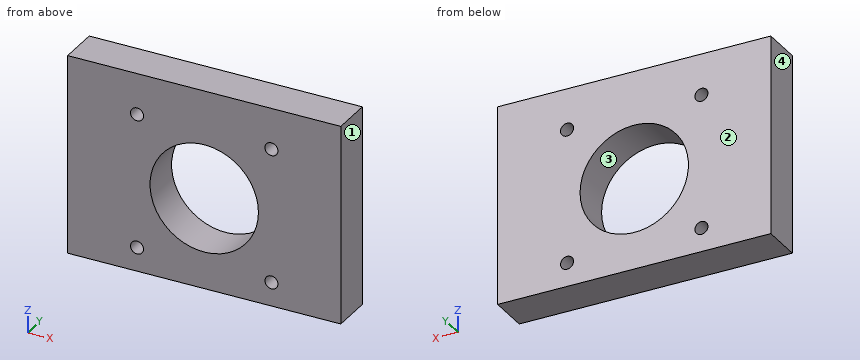
```python
from build123d import *

# Parameters (mm, degrees)
BOSS_EXTRUDE1_DEPTH = 46
CUT_EXTRUDE1_REACH  = 11.3
SKETCH2_R           = 12.5
SKETCH2_R_2         = 1.5


with BuildPart() as part:
    # Sketch1 → Boss-Extrude1 (new body)
    with BuildSketch(Plane.XY):
        Polygon((0, 0), (-31.5, 0), (-31.5, 9.3), (31.5, 9.3), (31.5, 0), align=None)
    extrude(amount=BOSS_EXTRUDE1_DEPTH)

    # Sketch2 → Cut-Extrude1 (cut, up to next)
    with BuildSketch(Plane(origin=(0, 9.3, 0), x_dir=(1, 0, 0), z_dir=(0, 1, 0)), mode=Mode.PRIVATE) as cut_extrude1_sk1:
        with Locations((0, -21)):
            Circle(SKETCH2_R)
    cut_extrude1_tool1 = extrude(cut_extrude1_sk1.sketch, amount=-CUT_EXTRUDE1_REACH, mode=Mode.PRIVATE) & part.part
    add(cut_extrude1_tool1.solids().sort_by_distance((0, 9.3, 21))[0], mode=Mode.SUBTRACT)
    # Sketch2 → Cut-Extrude1 (cut, up to next)
    with BuildSketch(Plane(origin=(0, 9.3, 0), x_dir=(1, 0, 0), z_dir=(0, 1, 0)), mode=Mode.PRIVATE) as cut_extrude1_sk2:
        with Locations((-15.5, -5.5)):
            Circle(SKETCH2_R_2)
    cut_extrude1_tool2 = extrude(cut_extrude1_sk2.sketch, amount=-CUT_EXTRUDE1_REACH, mode=Mode.PRIVATE) & part.part
    add(cut_extrude1_tool2.solids().sort_by_distance((-15.5, 9.3, 5.5))[0], mode=Mode.SUBTRACT)
    # Sketch2 → Cut-Extrude1 (cut, up to next)
    with BuildSketch(Plane(origin=(0, 9.3, 0), x_dir=(1, 0, 0), z_dir=(0, 1, 0)), mode=Mode.PRIVATE) as cut_extrude1_sk3:
        with Locations((-15.5, -36.5)):
            Circle(SKETCH2_R_2)
    cut_extrude1_tool3 = extrude(cut_extrude1_sk3.sketch, amount=-CUT_EXTRUDE1_REACH, mode=Mode.PRIVATE) & part.part
    add(cut_extrude1_tool3.solids().sort_by_distance((-15.5, 9.3, 36.5))[0], mode=Mode.SUBTRACT)
    # Sketch2 → Cut-Extrude1 (cut, up to next)
    with BuildSketch(Plane(origin=(0, 9.3, 0), x_dir=(1, 0, 0), z_dir=(0, 1, 0)), mode=Mode.PRIVATE) as cut_extrude1_sk4:
        with Locations((15.5, -5.5)):
            Circle(SKETCH2_R_2)
    cut_extrude1_tool4 = extrude(cut_extrude1_sk4.sketch, amount=-CUT_EXTRUDE1_REACH, mode=Mode.PRIVATE) & part.part
    add(cut_extrude1_tool4.solids().sort_by_distance((15.5, 9.3, 5.5))[0], mode=Mode.SUBTRACT)
    # Sketch2 → Cut-Extrude1 (cut, up to next)
    with BuildSketch(Plane(origin=(0, 9.3, 0), x_dir=(1, 0, 0), z_dir=(0, 1, 0)), mode=Mode.PRIVATE) as cut_extrude1_sk5:
        with Locations((15.5, -36.5)):
            Circle(SKETCH2_R_2)
    cut_extrude1_tool5 = extrude(cut_extrude1_sk5.sketch, amount=-CUT_EXTRUDE1_REACH, mode=Mode.PRIVATE) & part.part
    add(cut_extrude1_tool5.solids().sort_by_distance((15.5, 9.3, 36.5))[0], mode=Mode.SUBTRACT)


solid = part.part
```
CAD build for the part. Positions are in the model's coordinates, mm. Face numbers are marked on the shaded views. Round coordinates to 2 decimals unless told otherwise and drop trailing zeros. Order: outer loops, then holes, each group sorted by start corner. A loop starts at its lowest first (then second) coordinate and runs counter-clockwise, first axis right, second up.
Q1. Two-plate mould, pull along X, no slides. Class the marked faces 1, 2, 3 and 4: pulls with the +X half, pulls with the -X half, needs draft (parallel to the pull), parting line crosses it, or undercut.
Q2. Slice it at D-D (x = -10.5). Write the cut outline in (y, z).
Q3. Slice it at C-C (y = 2.5). Write the cut outline in (x, z).
Q4. Wall check: L1, parallel to Z at x = -15.5, y = 4.75; L2, parallel to X at y = 4, z = 5.5; L3, parallel to X at y = 4.75, z = 21. Give the ranges that are in metal, low to high.
Q5. Slice it at B-B (z = 5.5). Write the cut outline in (x, y).
Q6. Slice it at A-A (x = 15.5). Write the cut outline in (y, z), and give its area (3 significant figures).
Results below:
1. face 1: pulls with the +X half
1. face 2: needs draft
1. face 3: undercut
1. face 4: pulls with the -X half
2. outline: (0, 0) - (9.3, 0) - (9.3, 14.22) - (0, 14.22) - close; (0, 27.78) - (9.3, 27.78) - (9.3, 46) - (0, 46) - close
3. outline: (-31.5, 0) - (31.5, 0) - (31.5, 46) - (-31.5, 46) - close; hole circle Ø3 at (-15.5, 5.5); hole circle Ø3 at (-15.5, 36.5); hole circle Ø25 at (0, 21); hole circle Ø3 at (15.5, 5.5); hole circle Ø3 at (15.5, 36.5)
4. L1: z = 0 to 4, 7 to 35, 38 to 46
4. L2: x = -31.5 to -17, -14 to 14, 17 to 31.5
4. L3: x = -31.5 to -12.5, 12.5 to 31.5
5. outline: (-31.5, 0) - (-17, 0) - (-17, 9.3) - (-31.5, 9.3) - close; (-14, 0) - (14, 0) - (14, 9.3) - (-14, 9.3) - close; (17, 0) - (31.5, 0) - (31.5, 9.3) - (17, 9.3) - close
6. outline: (0, 0) - (9.3, 0) - (9.3, 4) - (0, 4) - close; (0, 7) - (9.3, 7) - (9.3, 35) - (0, 35) - close; (0, 38) - (9.3, 38) - (9.3, 46) - (0, 46) - close
6. area: 372 mm2
